from build123d import *

# Parameters (mm, degrees)
SKIZZE1_W                       = 150
SKIZZE1_H                       = 100
AUFSATZ_LINEAR_AUSTRAGEN1_DEPTH = 50
SKIZZE2_W                       = 100
SKIZZE2_H                       = 80
SCHNITT_LINEAR_AUSTRAGEN1_DEPTH = 5
SKIZZE3_W                       = 50
SKIZZE3_H                       = 50
AUFSATZ_LINEAR_AUSTRAGEN2_DEPTH = 2.5
SKIZZE4_R                       = 5
SCHNITT_LINEAR_AUSTRAGEN2_DEPTH = 10
VERRUNDUNG1_SIZE                = 50
VERRUNDUNG1_SIZE_2              = 40
SKIZZE5_R                       = 5
SCHNITT_LINEAR_AUSTRAGEN3_DEPTH = 380


with BuildPart() as part:
    # Skizze1 → Aufsatz-Linear austragen1 (new body)
    with BuildSketch(Plane(origin=(0, 0, 0), x_dir=(0, 0, -1), z_dir=(1, 0, 0))):
        with Locations((-31.954225352, -9.463028169)):
            Rectangle(SKIZZE1_W, SKIZZE1_H)
    extrude(amount=AUFSATZ_LINEAR_AUSTRAGEN1_DEPTH)

    # Skizze2 → Schnitt-Linear austragen1 (cut)
    with BuildSketch(Plane(origin=(50, 0, 0), x_dir=(0, 0, -1), z_dir=(1, 0, 0))):
        with Locations((-6.954225352, -19.463028169)):
            Rectangle(SKIZZE2_W, SKIZZE2_H)
    extrude(amount=-SCHNITT_LINEAR_AUSTRAGEN1_DEPTH, mode=Mode.SUBTRACT)

    # Skizze3 → Aufsatz-Linear austragen2 (add)
    with BuildSketch(Plane(origin=(45, 0, 0), x_dir=(0, 0, -1), z_dir=(1, 0, 0))):
        with Locations((18.045774648, -19.463028169)):
            Rectangle(SKIZZE3_W, SKIZZE3_H)
    extrude(amount=AUFSATZ_LINEAR_AUSTRAGEN2_DEPTH)

    # Skizze4 → Schnitt-Linear austragen2 (cut)
    with BuildSketch(Plane(origin=(47.5, 0, 0), x_dir=(0, 0, -1), z_dir=(1, 0, 0))):
        with Locations((33.045774648, -19.463028169)):
            Circle(SKIZZE4_R)
        with Locations((13.045774648, -19.463028169)):
            Circle(SKIZZE4_R)
    extrude(amount=-SCHNITT_LINEAR_AUSTRAGEN2_DEPTH, mode=Mode.SUBTRACT)

    # Verrundung1
    # an asymmetric fillet: 50, 40 mm, written as the material it takes off along each edge
    with BuildSketch(Plane(origin=(-125, -59.463028169, 106.954225352), x_dir=(0, 1, 0), z_dir=(1, 0, 0))) as verrundung1_piece_1:
        with BuildLine():
            Bezier((VERRUNDUNG1_SIZE, 0), (0, 0), (0, -VERRUNDUNG1_SIZE_2), weights=[1, 0.707106781, 1])
            Line((0, -VERRUNDUNG1_SIZE_2), (0, 0))
            Line((0, 0), (VERRUNDUNG1_SIZE, 0))
        make_face()
    extrude(amount=300, mode=Mode.SUBTRACT)
    with BuildSketch(Plane(origin=(-125, 40.536971831, 106.954225352), x_dir=(0, 0, -1), z_dir=(1, 0, 0))) as verrundung1_piece_2:
        with BuildLine():
            Bezier((VERRUNDUNG1_SIZE_2, 0), (0, 0), (0, -VERRUNDUNG1_SIZE), weights=[1, 0.707106781, 1])
            Line((0, -VERRUNDUNG1_SIZE), (0, 0))
            Line((0, 0), (VERRUNDUNG1_SIZE_2, 0))
        make_face()
    extrude(amount=300, mode=Mode.SUBTRACT)

    # Skizze5 → Schnitt-Linear austragen3 (cut)
    with BuildSketch(Plane.ZY):
        with Locations((85.614751131, -9.463028169)):
            Circle(SKIZZE5_R)
    extrude(amount=-SCHNITT_LINEAR_AUSTRAGEN3_DEPTH, mode=Mode.SUBTRACT)


solid = part.part
For this review, take the finished solid that the model builds, in its own axes (mm). A direction names the side the tool comes from. Coordinates: 2 decimals unless noted, no trailing zeros. Loops run counter-clockwise (first coordinate to the right, second up) from the corner with the lowest first, then second, coordinate; pieces in that order, holes last. Notation, with made-up numbers: (85.25, -12.75) -> (123.25, -12.75) arc R20 ccw to (123.25, 21.25) -> close; hole circle Ø10 at (85, 59). An arc over 180 degrees is marked (long way). Write each question's results on one line, items separated by ' | '.
Q1. Machinability: for faces 1 (the flat face through (48, -20, 56.954)), 2 (the flat face through (37.5, -19, -33)), 3 (the flat face through (47.5, -25, -18)), which of the approach directions +Z, -Z, +X, -X, +Y, -Y give a long, thin tool a straight path to every point of the face, cutting with its end or side? Answer none if there is none.
Taken from the geometry:
face 1: +X, -Y | face 2: +X | face 3: -Z, +X, -Y
Q2. Add section A-A, the plane z = 46. State the section outline as (x, y) points, then the cut area to 3 significant figures.
Taken from the geometry:
outline: (0, -59.46) -> (45, -59.46) -> (45, 20.54) -> (50, 20.54) -> (50, 40.54) -> (0, 40.54) -> close | area: 4,600 mm²
Q3. For pin 1 Ø3 at (y, z) = (-20.5, -14) entering from +X; pin 2 Ø3 at (y, z) = (-39.5, 85.5) entering from -X; pin 3 Ø2 at (y, z) = (-14, 40) entering from +X; pin 4 Ø8 at (x, z) = (9.5, 86) entering from +Y (3 decimals), all flat-tipped, find the tip position at first contact; note any pin that passes through.
Taken from the geometry:
pin 1: x = 37.5 | pin 2: x = 0 | pin 3: x = 45 | pin 4: y = 36.865
Q4. To check wall thickness, follow line 1 along Z through (x, y) = (16, -10); line 2 along X through (y, z) = (-13, -13); line 3 along Y through (x, z) = (20.5, 81.5). State the ranges of each line that lie inside material, in increasing order. Write a range as [from, to].
Taken from the geometry:
line 1: [-43.05, 80.64], [90.59, 106.95] | line 2: [0, 47.5] | line 3: [-56.04, -12.3], [-6.62, 37.11]
Q5. Add section B-B, the plane z = -30. State the section outline as (x, y) points.
Taken from the geometry:
outline: (0, -59.46) -> (45, -59.46) -> (45, -44.46) -> (47.5, -44.46) -> (47.5, -23.43) -> (37.5, -23.43) -> (37.5, -15.5) -> (47.5, -15.5) -> (47.5, 5.54) -> (45, 5.54) -> (45, 20.54) -> (50, 20.54) -> (50, 40.54) -> (0, 40.54) -> close
Q6. Mouldability with a two-part tool opening along Y and no side actions: class faces 4 (the flat face through (25, 40.537, 13)), 5 (the cylindrical face through (42.57, -21.378, -37.665)), 6 (the flat face through (25, -59.463, 13)) as +Y half, -Y half, draft (parallel to the pull), parting line (faces both ways), or undercut.
Taken from the geometry:
face 4: +Y half | face 5: undercut | face 6: -Y half
